Could you check a few things on this model? Use its own coordinates, in mm. A direction names the side the tool comes from. Give positions to 0.01 mm unless a question says otherwise; leave off trailing zeros. Loops run counter-clockwise (first coordinate to the right, second up) from the corner with the lowest first, then second, coordinate; pieces in that order, holes last. Notation, with made-up numbers: M -21,72 L -6,72 A22 cw -6,96 Z; hole C 20,-29.5 d2. An arc over 180 degrees is marked long. Write each question's results on one line, items separated by ' | '. Start each with the question number.
from build123d import *

# Parameters (mm, degrees)
F1_DEPTH = 5
F2_SIZE  = 0.5
F3_R     = 4
F4_DEPTH = 65
F5_R     = 2


with BuildPart() as f1:
    # F0 (on Front) → F1 (new body)
    with BuildSketch(Plane.XZ):
        Polygon((0, 6.9282032303), (-6, 3.4641016151), (-6, 0), (-6, -3.4641016151), (0, -6.9282032303), (3, -5.1961524227), (6, -3.4641016151), (6, 0), (6, 3.4641016151), (3, 5.1961524227), align=None)
    extrude(amount=-F1_DEPTH)

    # F2
    f2_edges = [f1.edges().sort_by_distance(p)[0] for p in [
        (-3, 5, 5.196152),
        (-6, 5, 0),
        (-3, 5, -5.196152),
        (3, 5, -5.196152),
        (6, 5, 0),
        (3, 5, 5.196152),
    ]]
    chamfer(f2_edges, length=F2_SIZE)

    # F3 (on face) → F4 (join)
    with BuildSketch(Plane.XZ):
        Circle(F3_R)
    extrude(amount=F4_DEPTH)

    # F5
    f5_edges = [f1.edges().sort_by_distance(p)[0] for p in [
        (-4, -65, 0),
    ]]
    fillet(f5_edges, radius=F5_R)


solid = f1.part
1) If we section it at A-A on y = -30.5: Write out the boundary of the cut face in (x, z).
2) Please list where these lines run through material, in increasing order: line 1 (Y direction, x = -4.75, z = 3); line 2 (Z direction, x = 0.25, y = -16); line 3 (Z direction, x = 1.5, y = -1). Write a range as from..to.
3) Which directions (+Z, -Z, +X, -X, +Y, -Y) give clear straight access to the entire face, cutting with the end or side of a thin tool? Please do faces 1 (the face through (-3, 0, -3)), 2 (the face through (0, 5, 0)).
4) If we section it at B-B on z = 5: Write out the boundary of the cut face in (x, y).
5) I'm going to push flat-ended pins straight in: P1, Ø5, axis at x = 1.5, y = -28, coming from the -Z side; P2, Ø6, axis at y = -8.5, z = -2, coming from the -X side; P3, Ø8, axis at y = -52.5, z = 2, coming from the +X side. Where does each tip first touch, or does it pass through?
Calculated:
1) outline: C 0,0 d8
2) line 1: y = 0..5 | line 2: z = -3.99..3.99 | line 3: z = -3.71..3.71
3) face 1: -Y | face 2: +Z, -Z, +X, -X, +Y
4) outline: M -3.34,0 L 3.34,0 L 3.34,4.5 L 2.34,5 L -2.34,5 L -3.34,4.5 Z
5) P1: stops at z = -4 | P2: stops at x = -4 | P3: stops at x = 4
